Part model, mm, in its own coordinate system. A direction names the side the tool comes from. Round coordinates to 2 decimals unless told otherwise and drop trailing zeros. Loops run counter-clockwise (first coordinate to the right, second up) from the corner with the lowest first, then second, coordinate; pieces in that order, holes last.
1) Drop flat-ended pins along their axis: P1, Ø1.5, axis at x = -13, z = -2.5, coming from the -Y side; P2, Ø10.5, axis at x = 31.5, z = -9, coming from the -Y side; P3, Ø6, axis at y = -14, z = -6.5, coming from the +X side. Give the stop position or say it passes through.
2) Band-saw the part on D-D, the plane x = 29. Write the cut outline in (y, z).
3) Band-saw the part on B-B, the plane x = -26. Write the cut outline in (y, z), then the cut area to 3 significant figures.
4) 3-axis set-ups, long thin cutter, end or side, ignore diameter. For faces 5 (the flat face through (0, -24, 15)), 6 (the flat face through (-30, -3, 9)), 7 (the cylindrical face through (-0.495, -22.495, 0.196)), 8 (the flat face through (26, -10, -5)), 9 (the flat face through (-26, -10, -5)): which of +Z, -Z, +X, -X, +Y, -Y reach the whole face in a straight line?
5) Mould opens along X. For faces 1 (the cylindrical face through (-35, -9, 0)), 2 (the cylindrical face through (35, -9, 0)), 3 (the flat face through (-25.323, -9, 0)), 4 (the flat face through (30, -3, 9)) say: +X half, -X half, draft (parallel to the pull), parting line (faces both ways), or undercut.
6) Band-saw the part on C-C, the plane y = -9. State how many separate pieces and enclosed holes the cut face has, then the cut area to 3 significant figures.
7) Band-saw the part on A-A, the plane z = 7.5. Write the cut outline in (x, y).
8) Probe line 1 (Z direction, x = 30, y = -1.9); line 2 (X direction, y = -5, z = 0) (3 decimals); line 3 (X direction, y = -9.25, z = 0). List the from-to ranges inside material, lowest first.
from build123d import *

# Parameters (mm, degrees)
BOSS_EXTRUDE1_DEPTH       = 15
BOSS_EXTRUDE2_START       = -5
BOSS_EXTRUDE2_DEPTH       = 10
BOSS_EXTRUDE2_START_2     = -15
BOSS_EXTRUDE2_2_DEPTH     = 12
BOSS_EXTRUDE2_3_OUTLINE_R = 3
BOSS_EXTRUDE2_3_DEPTH     = 12
BOSS_EXTRUDE2_START_3     = -3
BOSS_EXTRUDE2_4_DEPTH     = 6
FILLET1_R                 = 1
SKETCH4_4_R               = 3
CUT_EXTRUDE1_DEPTH        = 45.229515196
SKETCH5_R                 = 3
CUT_EXTRUDE2_DEPTH        = 41.926764018


with BuildPart() as part:
    # Sketch2 → Boss-Extrude1 (new, symmetric)
    with BuildSketch(Plane.XY):
        with BuildLine():
            Line((-35, 0), (-22.5, 0))
            ThreePointArc((-22.5, 0), (0, -22.5), (22.5, 0))
            Line((22.5, 0), (35, 0))
            Line((35, 0), (35, -3))
            Line((35, -3), (25.322914524, -3))
            ThreePointArc((25.322914524, -3), (0, -25.5), (-25.322914524, -3))
            Line((-25.322914524, -3), (-35, -3))
            Line((-35, -3), (-35, 0))
        make_face()
    extrude(amount=BOSS_EXTRUDE1_DEPTH, both=True)

    # Boss-Extrude2: read off the stored shape, not the designer's step
    # Boss-Extrude2 outline → Boss-Extrude2 (add)
    with BuildSketch(Plane.XY.offset(BOSS_EXTRUDE2_START)):
        with BuildLine():
            Line((25.322914524, -15), (25.322914524, -3))
            ThreePointArc((25.322914524, -3), (23.742880794, -9.301914405), (20.621590627, -15))
            Line((20.621590627, -15), (25.322914524, -15))
        make_face()
    boss_extrude2 = extrude(amount=BOSS_EXTRUDE2_DEPTH)

    # Boss-Extrude2 2 outline → Boss-Extrude2 2 (cut)
    with BuildSketch(Plane(origin=(0, 0, 0), x_dir=(1, 0, 0), z_dir=(0, 1, 0)).offset(BOSS_EXTRUDE2_START_2)):
        with BuildLine():
            Line((25.322914524, -1.767730594), (25.322914524, 1.767730594))
            ThreePointArc((25.322914524, 1.767730594), (25, 0), (25.322914524, -1.767730594))
        make_face()
    boss_extrude2_2 = extrude(amount=BOSS_EXTRUDE2_2_DEPTH, mode=Mode.SUBTRACT)

    # Boss-Extrude2 3 outline → Boss-Extrude2 3 (add)
    with BuildSketch(Plane(origin=(0, 0, 0), x_dir=(1, 0, 0), z_dir=(0, 1, 0)).offset(BOSS_EXTRUDE2_START_2)):
        with BuildLine():
            ThreePointArc((30, -5), (35, 0), (30, 5))
            Line((30, 5), (25.322914524, 5))
            Line((25.322914524, 5), (25.322914524, -5))
            Line((25.322914524, -5), (30, -5))
        make_face()
        with Locations((30, 0)):
            Circle(BOSS_EXTRUDE2_3_OUTLINE_R, mode=Mode.SUBTRACT)
    boss_extrude2_3 = extrude(amount=BOSS_EXTRUDE2_3_DEPTH)

    # Boss-Extrude2 4 outline → Boss-Extrude2 4 (add)
    with BuildSketch(Plane.XY.offset(BOSS_EXTRUDE2_START_3)):
        with BuildLine():
            ThreePointArc((24.999860048, -5.025634049), (25.181763411, -4.016066673), (25.322914524, -3))
            Line((25.322914524, -3), (24, -3))
            Line((24, -3), (24, -7))
            Line((24, -7), (24.602960196, -7))
            Line((24.602960196, -7), (24.999860048, -5.025634049))
        make_face()
    boss_extrude2_4 = extrude(amount=BOSS_EXTRUDE2_4_DEPTH)

    # Fillet1
    fillet1_edges = [part.edges().sort_by_distance(p)[0] for p in [
        (30.161457262, -3, -15),
        (0, -25.5, -15),
        (-30.161457262, -3, -15),
        (-35, -1.5, -15),
        (0, -25.5, 15),
        (30.161457262, -3, 15),
        (35, -1.5, 15),
        (28.75, 0, 15),
        (0, -22.5, 15),
        (-28.75, 0, 15),
        (-35, -1.5, 15),
        (-28.75, 0, -15),
        (-30.161457262, -3, 15),
        (0, -22.5, -15),
        (28.75, 0, -15),
        (35, -1.5, -15),
    ]]
    fillet(fillet1_edges, radius=FILLET1_R)

    # Sketch4_4 → Cut-Extrude1 (cut, through all)
    with BuildSketch(Plane.XZ.offset(3)):
        with Locations(Location((30, 0, 0), (0, 0, 270))):
            Circle(SKETCH4_4_R)
    extrude(amount=-CUT_EXTRUDE1_DEPTH, mode=Mode.SUBTRACT)

    # Mirror1: Boss-Extrude2, Boss-Extrude2 2, Boss-Extrude2 3, Boss-Extrude2 4 across plane
    add(boss_extrude2.mirror(Plane(origin=(0, 0, 0), x_dir=(0, 0, 1), z_dir=(1, 0, 0))))
    add(boss_extrude2_2.mirror(Plane(origin=(0, 0, 0), x_dir=(0, 0, 1), z_dir=(1, 0, 0))), mode=Mode.SUBTRACT)
    add(boss_extrude2_3.mirror(Plane(origin=(0, 0, 0), x_dir=(0, 0, 1), z_dir=(1, 0, 0))))
    add(boss_extrude2_4.mirror(Plane(origin=(0, 0, 0), x_dir=(0, 0, 1), z_dir=(1, 0, 0))))

    # Sketch5 → Cut-Extrude2 (cut, through all)
    with BuildSketch(Plane.XZ.offset(15)):
        with Locations(Location((-30, 0, 0), (0, 0, 270))):
            Circle(SKETCH5_R)
    extrude(amount=-CUT_EXTRUDE2_DEPTH, mode=Mode.SUBTRACT)


solid = part.part
Reported:
1. P1: stops at y = -22.36
1. P2: stops at y = -15
1. P3: stops at x = 33.57
2. outline: (-15, -5) - (-3, -5) - (-3, -14) arc R1 ccw to (-2, -15) - (-1, -15) arc R1 ccw to (0, -14) - (0, -2.83) - (-15, -2.83) - close; (-15, 2.83) - (0, 2.83) - (0, 14) arc R1 ccw to (-1, 15) - (-2, 15) arc R1 ccw to (-3, 14) - (-3, 5) - (-15, 5) - close
3. outline: (-15, -5) - (-3, -5) - (-3, -14) arc R1 ccw to (-2, -15) - (-1, -15) arc R1 ccw to (0, -14) - (0, 14) arc R1 ccw to (-1, 15) - (-2, 15) arc R1 ccw to (-3, 14) - (-3, 5) - (-15, 5) - close
3. area: 209 mm2
4. face 5: +Z, +X, -X, +Y, -Y
4. face 6: +Z, -X, -Y
4. face 7: +Z, -Z, +Y
4. face 8: -Z, +X, -Y
4. face 9: -Z, -X, -Y
5. face 1: -X half
5. face 2: +X half
5. face 3: undercut
5. face 4: draft
6. separate pieces: 2
6. enclosed holes: 4
6. area: 336 mm2
7. outline: (-35, -3) - (-25.32, -3) arc R25.5 ccw to (25.32, -3) - (35, -3) - (35, 0) - (22.5, 0) arc R22.5 cw to (-22.5, 0) - (-35, 0) - close
8. line 1: z = -15 to -3, 3 to 15
8. line 2: x = -35 to -33, -27 to -25.323, -25.005 to -21.937, 21.937 to 25.005, 25.323 to 27, 33 to 35
8. line 3: x = -35 to -33, -27 to -25.32, -25 to -20.51, 20.51 to 25, 25.32 to 27, 33 to 35
